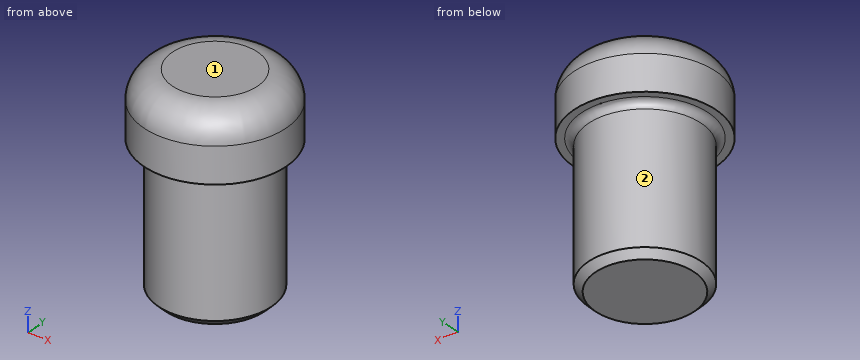
from build123d import *

# Parameters (mm, degrees)
SKETCH1_R           = 3.975
BOSS_EXTRUDE1_DEPTH = 10
SKETCH2_R           = 5
BOSS_EXTRUDE2_DEPTH = 4.5
FILLET4_R           = 2
FILLET5_R           = 0.5
CHAMFER1_SIZE       = 0.5


with BuildPart() as part:
    # Sketch1 → Boss-Extrude1 (new body)
    with BuildSketch(Plane.XY):
        Circle(SKETCH1_R)
    extrude(amount=BOSS_EXTRUDE1_DEPTH)

    # Sketch2 → Boss-Extrude2 (add)
    with BuildSketch(Plane.XY.offset(10)):
        Circle(SKETCH2_R)
    extrude(amount=BOSS_EXTRUDE2_DEPTH)

    # Fillet4
    fillet4_edges = [part.edges().sort_by_distance(p)[0] for p in [
        (-5, 0, 14.5),
    ]]
    fillet(fillet4_edges, radius=FILLET4_R)

    # Fillet5
    fillet5_edges = [part.edges().sort_by_distance(p)[0] for p in [
        (-3.975, 0, 10),
    ]]
    fillet(fillet5_edges, radius=FILLET5_R)

    # Chamfer1
    chamfer1_edges = [part.edges().sort_by_distance(p)[0] for p in [
        (-3.975, 0, 0),
    ]]
    chamfer(chamfer1_edges, length=CHAMFER1_SIZE)


solid = part.part
Geometry: final body of the model. Coordinates: model frame, mm. Face numbers are marked on the shaded views. A direction names the side the tool comes from. Round coordinates to 2 decimals unless told otherwise and drop trailing zeros. Order: outer loops, then holes, each group sorted by start corner. A loop starts at its lowest first (then second) coordinate and runs counter-clockwise, first axis right, second up. Notation, with made-up numbers: (73, 9.5) -> (80, 9.5) arc R24 ccw to (80, 38.5) -> close; hole circle Ø7 at (-28, 28). An arc over 180 degrees is marked (long way). Put each result on its own line as item: value. Start each with the question number.
Q1. Line query: probe 1 along Y at (x, z) = (0, 6.5) (3 decimals); probe 2 along Z at (x, y) = (-4.25, 1); probe 3 along X at (y, z) = (2.5, 13.5). Output: solid intervals per line, ascending.
Q2. First-contact query: pin 1 (1.5 mm diameter, centred on x = 3.5, z = 11, fed in from -Y); pin 2 (3 mm diameter, centred on x = -0.5, y = 1.5, fed in from -Z); pin 3 (1.5 mm diameter, centred on y = 4, z = 7.5, fed in from +X); pin 4 (1.5 mm diameter, centred on y = -3.5, z = 3, fed in from -X). Flat tips, straight axial feed; report the tip coordinate or a pass-through.
Q3. Section D-D on z = 10.75. Return the cut outline in (x, y).
Q4. Section A-A on x = 0. Return the cut outline in (y, z) (3 decimals).
Q5. Reachability of the marked faces 1 and 2 from +Z, -Z, +X, -X, +Y, -Y: full face, straight path, thin tool, end or side. Return the list, or none.
Q6. Section C-C on z = 4.5. Return the cut outline in (x, y) (3 decimals), and give its area (3 significant figures).
Ans:
1. probe 1: y = -3.975 to 3.975
1. probe 2: z = 9.99 to 13.96
1. probe 3: x = -4.02 to 4.02
2. pin 1: stops at y = -4.18
2. pin 2: stops at z = 0
2. pin 3: stops at x = 2.29
2. pin 4: stops at x = -2.87
3. outline: circle Ø10 at (0, 0)
4. outline: (-5, 10) -> (-4.475, 10) arc R0.5 cw to (-3.975, 9.5) -> (-3.975, 0.5) -> (-3.475, 0) -> (3.475, 0) -> (3.975, 0.5) -> (3.975, 9.5) arc R0.5 cw to (4.475, 10) -> (5, 10) -> (5, 12.5) arc R2 ccw to (3, 14.5) -> (-3, 14.5) arc R2 ccw to (-5, 12.5) -> close
5. face 1: +Z, +X, -X, +Y, -Y
5. face 2: -Z
6. outline: circle Ø7.95 at (0, 0)
6. area: 49.6 mm2
